The listing builds one solid part. Answer for the finished solid, in the listing's coordinates (mm). Round coordinates to 2 decimals unless told otherwise and drop trailing zeros. Write each loop counter-clockwise with the first axis right and the second up, starting at its lowest first coordinate (ties: lowest second). Pieces come first, ordered by that corner, then holes. Notation, with made-up numbers: (48, 82.25) - (91, 82.25) arc R13 ccw to (91, 104.25) - close; hole circle Ø9 at (69, -4). An arc over 180 degrees is marked (long way). Answer in a Markdown table with one row per item.
from build123d import *

# Parameters (mm, degrees)
SKETCH1_R           = 6.35
BOSS_EXTRUDE1_DEPTH = 6.35
SKETCH2_R           = 6.35
CUT_EXTRUDE1_DEPTH  = 6.35
CUT_EXTRUDE2_START  = -6.35
CUT_EXTRUDE2_DEPTH  = 6.35
SKETCH4_W           = 6.35
SKETCH4_H           = 19.05
BOSS_EXTRUDE2_DEPTH = 19.05
SKETCH5_W           = 12.7
SKETCH5_H           = 12.7
CUT_EXTRUDE3_DEPTH  = 19.05


with BuildPart() as part:
    # Sketch1 → Boss-Extrude1 (new body)
    with BuildSketch(Plane(origin=(0, 0, 0), x_dir=(1, 0, 0), z_dir=(0, 1, 0))):
        with BuildLine():
            Line((0, -9.525), (-567.5074248, -9.525))
            ThreePointArc((-567.5074248, -9.525), (-577.0324248, 0), (-567.5074248, 9.525))
            Line((-567.5074248, 9.525), (0, 9.525))
            ThreePointArc((0, 9.525), (9.525, 0), (0, -9.525))
        make_face()
        with Locations(Location((-567.5074248, 0, 0), (0, 0, 270))):
            Circle(SKETCH1_R, mode=Mode.SUBTRACT)
    extrude(amount=BOSS_EXTRUDE1_DEPTH)

    # Sketch2 → Cut-Extrude1 (cut)
    with BuildSketch(Plane(origin=(0, 6.35, 0), x_dir=(1, 0, 0), z_dir=(0, 1, 0))):
        with Locations(Location((-114.3, 0, 0), (0, 0, 270))):
            Circle(SKETCH2_R)
    extrude(amount=-CUT_EXTRUDE1_DEPTH, mode=Mode.SUBTRACT)

    # Sketch3 → Cut-Extrude2 (cut)
    with BuildSketch(Plane(origin=(0, 6.35, 0), x_dir=(1, 0, 0), z_dir=(0, 1, 0)).offset(CUT_EXTRUDE2_START)):
        with BuildLine():
            Line((0, -9.525), (0, 9.525))
            ThreePointArc((0, 9.525), (9.525, 0), (0, -9.525))
        make_face()
    extrude(amount=CUT_EXTRUDE2_DEPTH, mode=Mode.SUBTRACT)

    # Sketch4 → Boss-Extrude2 (add)
    with BuildSketch(Plane(origin=(0, 6.35, 0), x_dir=(1, 0, 0), z_dir=(0, 1, 0))):
        with Locations((-3.175, 0)):
            Rectangle(SKETCH4_W, SKETCH4_H)
    extrude(amount=BOSS_EXTRUDE2_DEPTH)

    # Sketch5 → Cut-Extrude3 (cut)
    with BuildSketch(Plane(origin=(0, 0, 0), x_dir=(0, 0, -1), z_dir=(1, 0, 0))):
        with Locations((0, 15.875)):
            Rectangle(SKETCH5_W, SKETCH5_H)
    extrude(amount=-CUT_EXTRUDE3_DEPTH, mode=Mode.SUBTRACT)


solid = part.part
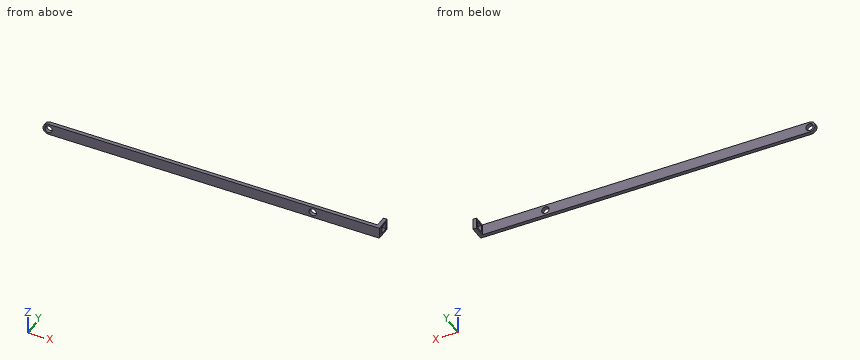
(1) Section C-C (x = -321) is taken. Give the vertices of the cut face in (y, z) (3 decimals).
Checked values:
| item | result |
|---|---|
| outline | (0, -9.525) - (6.35, -9.525) - (6.35, 9.525) - (0, 9.525) - close |
(2) Section B-B (z = 0) is taken. Give the vertices of the cut face in (x, y) (3 decimals), and give its area (3 significant figures).
Checked values:
| item | result |
|---|---|
| outline | (-577.032, 0) - (-573.857, 0) - (-573.857, 6.35) - (-577.032, 6.35) - close; (-561.157, 0) - (-120.65, 0) - (-120.65, 6.35) - (-561.157, 6.35) - close; (-107.95, 0) - (0, 0) - (0, 9.525) - (-6.35, 9.525) - (-6.35, 6.35) - (-107.95, 6.35) - close; (-6.35, 22.225) - (0, 22.225) - (0, 25.4) - (-6.35, 25.4) - close |
| area | 3,540 mm2 |
(3) Section A-A (x = -114.3) is taken. Give the vertices of the cut face in (y, z) (3 decimals).
Checked values:
| item | result |
|---|---|
| outline | (0, -9.525) - (6.35, -9.525) - (6.35, -6.35) - (0, -6.35) - close; (0, 6.35) - (6.35, 6.35) - (6.35, 9.525) - (0, 9.525) - close |
(4) Flat-ended cylindrical pins translate along their axes: pin 1 (10 mm diameter, centred on x = -444, z = 6, fed in from +Y); pin 2 (1.5 mm diameter, centred on x = -202, z = -4, fed in from -Y). Find the tip coordinate at first contact, or state that the pin passes through.
Checked values:
| item | result |
|---|---|
| pin 1 | stops at y = 6.35 |
| pin 2 | stops at y = 0 |
(5) Find the intervals of material crossed by line 1 (X direction, y = 3.75, z = 0); line 2 (X direction, y = 6.25, z = -3.25); line 3 (Y direction, x = -183, z = -7.75), in increasing order.
Checked values:
| item | result |
|---|---|
| line 1 | x = -577.03 to -573.86, -561.16 to -120.65, -107.95 to 0 |
| line 2 | x = -576.46 to -572.96, -562.05 to -119.76, -108.84 to 0 |
| line 3 | y = 0 to 6.35 |
